from build123d import *

# Parameters (mm, degrees)
F0_R     = 3
F1_DEPTH = 9
F3_D     = 5
F4_W     = 10
F4_H     = 18
F5_DEPTH = 3
F6_R     = 5
F7_SIZE  = 0.5


with BuildPart() as f1:
    # F0 (on Top) → F1 (new body)
    with BuildSketch(Plane.XY):
        Polygon((-5, -5.5), (5, -5.5), (5, 12.5), (14, 12.5), (14, 18), (-14, 18), (-14, 12.5), (-5, 12.5), align=None)
        Circle(F0_R, mode=Mode.SUBTRACT)
    extrude(amount=F1_DEPTH)

    # F3 (through all)
    with Locations(Plane.XZ.offset(-12.5)):
        with Locations((9, 4.5), (-9, 4.5)):
            Hole(F3_D / 2)

    # F4 (on face) → F5 (join)
    with BuildSketch(Plane.XY.offset(9)):
        with Locations((0, 3.5)):
            Rectangle(F4_W, F4_H)
    extrude(amount=F5_DEPTH)

    # F6
    f6_edges = [f1.edges().sort_by_distance(p)[0] for p in [
        (14, 15.25, 9),
        (-14, 15.25, 9),
    ]]
    fillet(f6_edges, radius=F6_R)

    # F7
    f7_edges = [f1.edges().sort_by_distance(p)[0] for p in [
        (-3, 0, 0),
        (5, 3.5, 0),
        (-5, 3.5, 0),
        (0, -5.5, 0),
        (-11.5, 12.5, 4.5),
        (6.5, 12.5, 4.5),
    ]]
    chamfer(f7_edges, length=F7_SIZE)


solid = f1.part
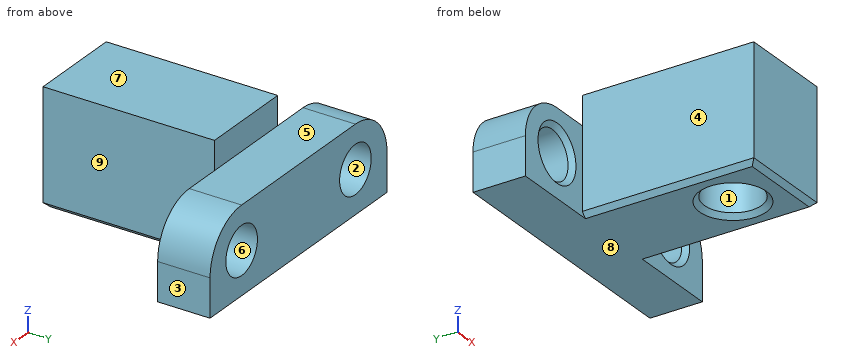
The listing builds one solid part. Answer for the finished solid, in the listing's coordinates (mm). Face numbers are marked on the shaded views. A direction names the side the tool comes from. Coordinates: 2 decimals unless noted, no trailing zeros. Write each loop counter-clockwise with the first axis right and the second up, starting at its lowest first coordinate (ties: lowest second). Pieces come first, ordered by that corner, then holes. Notation, with made-up numbers: (-18, 29.25) - (10, 29.25) arc R19 ccw to (10, 50.25) - close; hole circle Ø5 at (-27.75, 6.5). An arc over 180 degrees is marked (long way). Put each result on its own line as item: value.
1. The part is cut by section A-A on x = 0. Give the vertices of the cut face in (y, z).
Answer sheet:
outline: (-5.5, 0.5) - (-5, 0) - (-3.5, 0) - (-3, 0.5) - (-3, 9) - (3, 9) - (3, 0.5) - (3.5, 0) - (18, 0) - (18, 9) - (12.5, 9) - (12.5, 12) - (-5.5, 12) - close
2. Flat-ended cylindrical pins translate along their axes: pin 1 Ø2.5 at (x, z) = (-2, 11) entering from +Y; pin 2 Ø3 at (y, z) = (6, 6.5) entering from -X; pin 3 Ø2.5 at (x, z) = (-10.5, 4) entering from -Y. Find the tip coordinate at first contact, or state that the pin passes through.
Answer sheet:
pin 1: stops at y = 12.5
pin 2: stops at x = -5
pin 3: stops at y = 12.67
3. Find the intervals of material crossed by line 1 along Z through (x, y) = (9, 14.8); line 2 along Y through (x, z) = (0, 2.5); line 3 along Y through (x, z) = (5.25, 8.75), in increasing order. Write a range as from..to.
Answer sheet:
line 1: z = 0..2, 7..9
line 2: y = -5.5..-3, 3..18
line 3: y = 12.5..18
4. The part is cut by section D-D on z = 10.5. Give the vertices of the cut face in (x, y), plus the area to 3 significant figures.
Answer sheet:
outline: (-5, -5.5) - (5, -5.5) - (5, 12.5) - (-5, 12.5) - close
area: 180 mm^2
5. A tool of negligible diameter and unlimited length cuts with its end or side. For the marked faces 1, 2, 3, 4 and 5, from which of +Z, -Z, +X, -X, +Y, -Y can it reach the whole face along a straight path? Write none if from no direction.
Answer sheet:
face 1: -Z
face 2: +Y, -Y
face 3: +Z, -Z, +X, +Y, -Y
face 4: +Z, -Z, -X, -Y
face 5: +Z, +X, -X, +Y
6. The part is cut by section B-B on y = 0. Give the vertices of the cut face in (x, z), plus the area to 3 significant figures.
Answer sheet:
outline: (-5, 0.5) - (-4.5, 0) - (-3.5, 0) - (-3, 0.5) - (-3, 9) - (3, 9) - (3, 0.5) - (3.5, 0) - (4.5, 0) - (5, 0.5) - (5, 12) - (-5, 12) - close
area: 65.5 mm^2
7. Determine the mould class of the marked faces 6, 7, 8 and 9 for opening direction Z: pulls with the +Z half, pulls with the -Z half, needs draft (parallel to the pull), parting line crosses it, or undercut.
Answer sheet:
face 6: undercut
face 7: pulls with the +Z half
face 8: pulls with the -Z half
face 9: needs draft
8. The part is cut by section C-C on z = 5. State how many separate pieces and enclosed holes the cut face has, plus the area to 3 significant figures.
Answer sheet:
separate pieces: 3
enclosed holes: 1
area: 250 mm^2
